from build123d import *

# Parameters (mm, degrees)
SKETCH_2_R          = 1.585
CUT_EXTRUDE_1_DEPTH = 14


with BuildPart() as part:
    # 草图1 → 旋转1 (revolve)
    with BuildSketch(Plane.XY):
        Polygon((6.5, -3.25), (-6.5, -3.25), (-6.5, 3.25), (-5.5, 3.25), (-5.5, 1.25), (1, 1.25), (1, 3.25), (6.5, 3.25), align=None)
    revolve(axis=Axis((-6.5, -3.25, 0), (1, 0, 0)))

    # 草图2 → 切除-拉伸1 (cut, through all)
    with BuildSketch(Plane.ZY.offset(6.5)):
        with Locations((0, -3.25)):
            Circle(SKETCH_2_R)
    extrude(amount=-CUT_EXTRUDE_1_DEPTH, mode=Mode.SUBTRACT)


solid = part.part
Geometry check sheet. Reference: the model listing, model coordinates, mm. A direction names the side the tool comes from. Round coordinates to 2 decimals unless told otherwise and drop trailing zeros. Order: outer loops, then holes, each group sorted by start corner. A loop starts at its lowest first (then second) coordinate and runs counter-clockwise, first axis right, second up. Notation, with made-up numbers: (78.25, -38.75) -> (95.25, -38.75) arc R23 cw to (95.25, -26.75) -> close; hole circle Ø5 at (-7.75, 13.25). An arc over 180 degrees is marked (long way). Use one line per item in the form item = value.
1. Mould release check, pull along X, two halves, no side actions. Record for faces 3 (the face through (-5.5, 1, 2)), 4 (the face through (-2.204, 1.042, 1.352)), 5 (the face through (3.79, 2.95, 1.95)), 6 (the face through (6.5, -1.9, -1.4)): pulls with the +X half, pulls with the -X half, needs draft (parallel to the pull), parting line crosses it, or undercut.
Working result:
face_3 = undercut
face_4 = undercut
face_5 = needs draft
face_6 = pulls with the +X half
2. Cross-section at D-D, the plane z = 4. Enter the section's corners in (x, y), plus the area to 3 significant figures.
Working result:
outline = (-6.5, -8.37) -> (-5.5, -8.37) -> (-5.5, -5.31) -> (1, -5.31) -> (1, -8.37) -> (6.5, -8.37) -> (6.5, 1.87) -> (1, 1.87) -> (1, -1.19) -> (-5.5, -1.19) -> (-5.5, 1.87) -> (-6.5, 1.87) -> close
area = 93.4 mm^2
3. Cross-section at B-B, the plane z = 0. Enter the section's corners in (x, y) (3 decimals).
Working result:
outline = (-6.5, -9.75) -> (-5.5, -9.75) -> (-5.5, -7.75) -> (1, -7.75) -> (1, -9.75) -> (6.5, -9.75) -> (6.5, -4.835) -> (-6.5, -4.835) -> close; (-6.5, -1.665) -> (6.5, -1.665) -> (6.5, 3.25) -> (1, 3.25) -> (1, 1.25) -> (-5.5, 1.25) -> (-5.5, 3.25) -> (-6.5, 3.25) -> close
4. Set-up check for faces 1 (the face through (-5.99, 2.95, 1.95)), 2 (the face through (1, 1.2, -1.4)): record each of +Z, -Z, +X, -X, +Y, -Y from which the full face is reachable in a straight line by a thin tool's end or side.
Working result:
face_1 = +X, -X
face_2 = none
5. Go/stop test with flat-tipped pins: pin 1 (5 mm diameter, centred on x = -2.5, z = -1, fed in from +Y); pin 2 (1 mm diameter, centred on x = -2, z = 2.5, fed in from -Y); pin 3 (5 mm diameter, centred on x = -5, y = -7, fed in from +Z). Record where each tip stops, or that it passes through.
Working result:
pin_1 = 1.25
pin_2 = -7.28
pin_3 = 6.37
6. Cross-section at A-A, the plane y = -3.25. Enter the section's corners in (x, z) (3 decimals).
Working result:
outline = (-6.5, -6.5) -> (-5.5, -6.5) -> (-5.5, -4.5) -> (1, -4.5) -> (1, -6.5) -> (6.5, -6.5) -> (6.5, -1.585) -> (-6.5, -1.585) -> close; (-6.5, 1.585) -> (6.5, 1.585) -> (6.5, 6.5) -> (1, 6.5) -> (1, 4.5) -> (-5.5, 4.5) -> (-5.5, 6.5) -> (-6.5, 6.5) -> close
7. Cross-section at C-C, the plane x = 1.75. Enter the section's corners in (y, z) (3 decimals), plus the area to 3 significant figures.
Working result:
outline = circle Ø13 at (-3.25, 0); hole circle Ø3.17 at (-3.25, 0)
area = 125 mm^2
8. Scan lines: line 1 along X through (y, z) = (-5.75, 4.25); line 2 along Y through (x, z) = (4.25, -1.25); line 3 along Z through (x, y) = (0.5, -4.5). Record each from-to range of solid material in increasing order. Write a range as from..to.
Working result:
line_1 = -6.5..-5.5, 1..6.5
line_2 = -9.63..-4.22, -2.28..3.13
line_3 = -4.32..-0.97, 0.97..4.32
